Check sheet for the modelled part. Datum: model origin and axes. Units: mm. Coordinates: 2 decimals unless noted, no trailing zeros. Loops run counter-clockwise (first coordinate to the right, second up) from the corner with the lowest first, then second, coordinate; pieces in that order, holes last. Notation, with made-up numbers: (-21.75, 60.5) - (-7.75, 60.5) arc R10 ccw to (-7.75, 73.5) - close; hole circle Ø9 at (65, 47.25). An arc over 180 degrees is marked (long way). Use a Markdown table: item, result. Add a question column.
1) Thickness scan on line 1 (X direction, y = 0.25, z = 4); line 2 (Y direction, x = 2.5, z = -0.75); line 3 (X direction, y = -0.5, z = -2.5). Record the ranges inside material, lowest first.
2) Sectioned sample at A-A, the plane x = -100.5. Enter the section's corners in (y, z), then the cut area to 3 significant figures.
3) Go/stop test with flat-tipped pins: P1, Ø4, axis at x = -74, y = -4.5, coming from the -Z side; P2, Ø1, axis at x = -17, y = 2.5, coming from the -Z side; P3, Ø3, axis at x = -155.575, y = 0, coming from the +Z side. Record where each tip stops, or that it passes through.
from build123d import *

# Parameters (mm, degrees)
SKETCH1_R               = 6.35
BOSS_EXTRUDE1_DEPTH     = 163.5125
CHAMFER1_SIZE           = 1.5875
SKETCH2_R               = 1.984375
CUT_EXTRUDE1_DEPTH      = 7.35
CUT_EXTRUDE1_DEPTH_BACK = 7.35


with BuildPart() as part:
    # Sketch1 → Boss-Extrude1 (new body, symmetric)
    with BuildSketch(Plane(origin=(0, 0, 0), x_dir=(0, 0, -1), z_dir=(1, 0, 0))):
        Circle(SKETCH1_R)
    extrude(amount=BOSS_EXTRUDE1_DEPTH, both=True)

    # Chamfer1
    chamfer1_edges = [part.edges().sort_by_distance(p)[0] for p in [
        (-163.5125, 0, 6.35),
        (163.5125, 0, 6.35),
    ]]
    chamfer(chamfer1_edges, length=CHAMFER1_SIZE)

    # Sketch2 → Cut-Extrude1 (cut, two sides)
    with BuildSketch(Plane.XY) as cut_extrude1_sk:
        with Locations((-155.575, 0)):
            Circle(SKETCH2_R)
    extrude(amount=CUT_EXTRUDE1_DEPTH, mode=Mode.SUBTRACT)
    extrude(cut_extrude1_sk.sketch, amount=-CUT_EXTRUDE1_DEPTH_BACK, mode=Mode.SUBTRACT)


solid = part.part
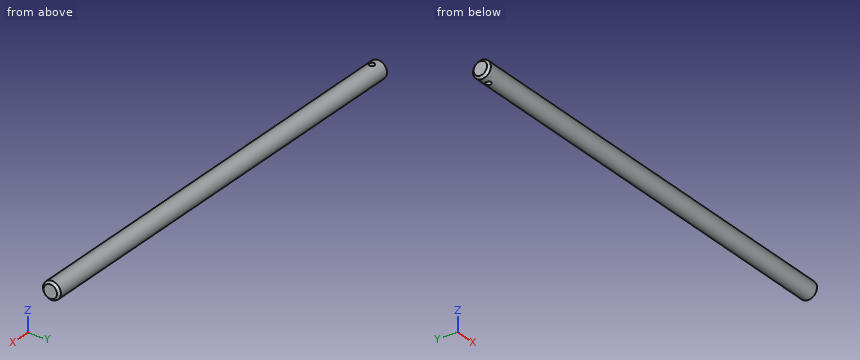
Solved:
| question | item | result |
|---|---|---|
| 1 | line 1 | x = -163.51 to -157.54, -153.61 to 163.51 |
| 1 | line 2 | y = -6.31 to 6.31 |
| 1 | line 3 | x = -163.51 to -157.5, -153.65 to 163.51 |
| 2 | outline | circle Ø12.7 at (0, 0) |
| 2 | area | 127 mm2 |
| 3 | P1 | stops at z = -5.84 |
| 3 | P2 | stops at z = -6.03 |
| 3 | P3 | passes through |
